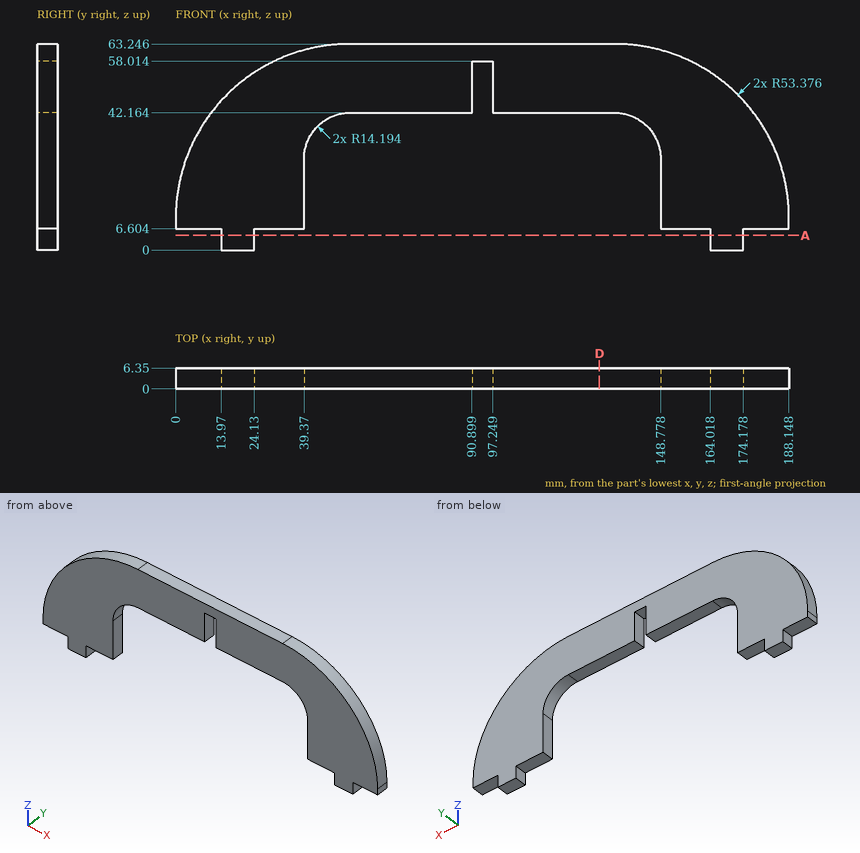
Print and shaded views of the part. All mm, measured from the part's lowest x, y and z. Coordinates: 2 decimals unless noted, no trailing zeros. Order: outer loops, then holes, each group sorted by start corner. A loop starts at its lowest first (then second) coordinate and runs counter-clockwise, first axis right, second up. Notation, with made-up numbers: (11.5, 42) -> (19.5, 42) arc R20 ccw to (19.5, 72) -> close; hole circle Ø1 at (-1.75, -13.5). An arc over 180 degrees is marked (long way). Answer as a JSON object with one key per item and string values. Group by question number.
1) Cut at A-A, the plane z = 4.5. Write the cut outline in (x, y).
2) Drill centre lines: L1, parallel to X at y = 2, z = 4.5; L2, parallel to X at y = 3, z = 11.5 (1 decimal); L3, parallel to Z at x = 55, y = 0.5. Where is each one in solid material? Low to high.
3) Cut at D-D, the plane x = 130. Write the cut outline in (y, z), then the cut area to 3 significant figures.
4) Flat gauge pins, fed straight in: pin 1 (3 mm diameter, centred on x = 8, y = 2, fed in from -Z); pin 2 (3 mm diameter, centred on x = 119.5, y = 3, fed in from -Z); pin 3 (10 mm diameter, centred on x = 86, z = 41, fed in from +Y); pin 4 (1 mm diameter, centred on x = 145.5, y = 4, fed in from +Z). Where does each tip first touch, or does it go through?
Check values:
{
 "1": {"outline": "(13.97, 0) -> (24.13, 0) -> (24.13, 6.35) -> (13.97, 6.35) -> close; (164.02, 0) -> (174.18, 0) -> (174.18, 6.35) -> (164.02, 6.35) -> close"},
 "2": {"L1": "x = 13.97 to 24.13, 164.02 to 174.18", "L2": "x = 0 to 39.4, 148.8 to 188.1", "L3": "z = 42.16 to 63.25"},
 "3": {"outline": "(0, 42.16) -> (6.35, 42.16) -> (6.35, 63.25) -> (0, 63.25) -> close", "area": "134 mm²"},
 "4": {"pin 1": "stops at z = 6.6", "pin 2": "stops at z = 42.16", "pin 3": "stops at y = 6.35", "pin 4": "stops at z = 62.26"}
}
